Autodesk Inventor part; units mm, degrees
ref_plane "YZ Plane" through (0, 0, 0) normal (1, 0, 0) x (0, 1, 0)
ref_plane "XZ Plane" through (0, 0, 0) normal (0, 1, 0) x (-1, 0, 0)
ref_plane "XY Plane" through (0, 0, 0) normal (0, 0, 1) x (1, 0, 0)
sketch "Sketch1" plane through (0, 0, 0) normal (0, 0, 1) x (1, 0, 0)
  line L0 (-3, 0) -> (-3, 88.9)
  line L1 (-3, 88.9) -> (0, 88.9)
  line L2 (0, 88.9) -> (0, 0)
  line L3 (-3, 0) -> (-4, 0)
  line L4 (-4, 0) -> (-4, -6)
  line L5 (-4, -6) -> (-3.5, -6)
  line L6 (-3.5, -6) -> (-3.5, -5)
  line L7 (-3.5, -5) -> (0, -5)
  line L8 (0, -5) -> (0, 0)
  dimension "d0" = 3
  dimension "d1" = 88.9
  dimension "d7" = 6
  dimension "d9" = 4
  dimension "d10" = 1
  dimension "d11" = 0.5
revolve "Revolution1" add sketch "Sketch1" angle 360 about axis through (0, 88.9, 0) along (0, -1, 0)
equation "\"BendRadius\" = Thickness"
equation "\"BendReliefWidth\" = Thickness"
equation "\"BendReliefDepth\" = 0.5 * Thickness"
equation "\"CornerReliefSize\" = 4 * Thickness"
equation "\"MinimumRemnant\" = 2 * Thickness"
equation "\"TransitionRadius\" = BendRadius"
equation "\"JacobiRadiusSize\" = BendRadius"
equation "\"GapSize\" = Thickness"
properties part number "Pusher.Pushrod" material "Stainless Steel"
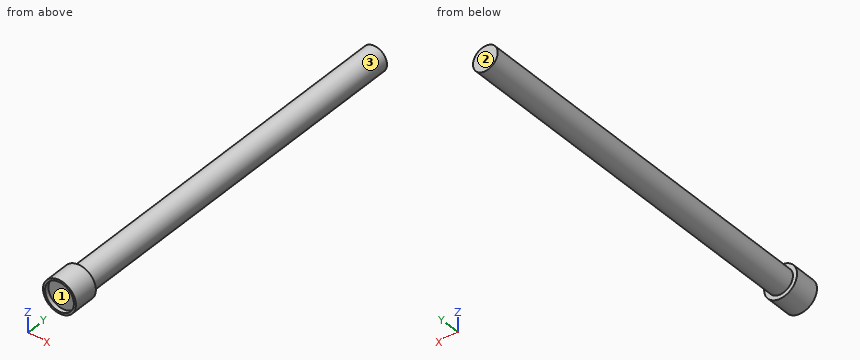
The model under review builds one solid part; all positions refer to its coordinate system, in mm. Face numbers are marked on the shaded views. Coordinates: 2 decimals unless noted, no trailing zeros. Order: outer loops, then holes, each group sorted by start corner. A loop starts at its lowest first (then second) coordinate and runs counter-clockwise, first axis right, second up. Notation, with made-up numbers: (5.5, 14) -> (36.5, 14) arc R11 cw to (36.5, 29) -> close; hole circle Ø8 at (44.25, 6). An arc over 180 degrees is marked (long way). Answer in a Markdown table with one row per item.
(1) Consider section B-B (x = 0). Write out the cut boundary in (y, z).
Answers:
| item | result |
|---|---|
| outline | (-6, -4) -> (0, -4) -> (0, -3) -> (88.9, -3) -> (88.9, 3) -> (0, 3) -> (0, 4) -> (-6, 4) -> (-6, 3.5) -> (-5, 3.5) -> (-5, -3.5) -> (-6, -3.5) -> close |
(2) Wall thickness on line 1 along Z through (x, y) = (0, -5.65); line 2 along Y through (x, z) = (0.75, 3.25): over which ranges is each line inside the solid? List them lowest first.
Answers:
| item | result |
|---|---|
| line 1 | -4 to -3.5, 3.5 to 4 |
| line 2 | -5 to 0 |
(3) The part is to be moulded in two halves that separate along X. For the marked faces 1, 2 and 3, say which applies: +X half, -X half, draft (parallel to the pull), parting line (faces both ways), or undercut.
Answers:
| item | result |
|---|---|
| face 1 | undercut |
| face 2 | draft |
| face 3 | parting line |
(4) Insertion check: pin 1 (1 mm diameter, centred on x = 2, y = 78, fed in from +Z); pin 2 (4 mm diameter, centred on x = 0, y = 39.5, fed in from +Z); pin 3 (1.5 mm diameter, centred on y = 74.5, z = 1, fed in from +X). Each pin has a flat end and moves straight along its axis. Give the tip position at first contact, or say it passes through.
Answers:
| item | result |
|---|---|
| pin 1 | z = 2.6 |
| pin 2 | z = 3 |
| pin 3 | x = 2.99 |
(5) Consider section A-A (z = 0). Write out the cut boundary in (x, y).
Answers:
| item | result |
|---|---|
| outline | (-4, -6) -> (-3.5, -6) -> (-3.5, -5) -> (3.5, -5) -> (3.5, -6) -> (4, -6) -> (4, 0) -> (3, 0) -> (3, 88.9) -> (-3, 88.9) -> (-3, 0) -> (-4, 0) -> close |
(6) Consider section C-C (y = 81). Write out the cut boundary in (x, z).
Answers:
| item | result |
|---|---|
| outline | circle Ø6 at (0, 0) |
